Geometry check sheet. Reference: the model listing, model coordinates, mm. A direction names the side the tool comes from. Coordinates: 2 decimals unless noted, no trailing zeros. Write each loop counter-clockwise with the first axis right and the second up, starting at its lowest first coordinate (ties: lowest second). Pieces come first, ordered by that corner, then holes. Notation, with made-up numbers: M 85,60 L 142,60 A12 cw 142,66 Z; hole C 49,79.25 d8. An arc over 180 degrees is marked long. Put each result on its own line as item: value. Start each with the question number.
1) Set-up check for faces 1 (the flat face through (20, 3, 52)), 2 (the flat face through (2, 0, -45)), 3 (the cylindrical face through (22.11, 16.76, 45.33)): record each of +Z, -Z, +X, -X, +Y, -Y from which the full face is reachable in a straight line by a thin tool's end or side.
2) Cross-section at D-D on y = 17.5. Record the cut outline in (x, z).
3) Gauge pin test, flat ends, axial feed: pin 1 (6 mm diameter, centred on x = 22.5, z = 44.5, fed in from -Y); pin 2 (4 mm diameter, centred on x = 29.5, z = -41.5, fed in from +Y); pin 3 (3 mm diameter, centred on x = 4, y = 0, fed in from -Z); pin 4 (7.5 mm diameter, centred on x = 16, y = 0, fed in from -Z). Record the tip position at first contact, or that the pin passes through.
4) Mould release check, pull along X, two halves, no side actions. Record for faces 4 (the flat face through (16, 14, -40)), 5 (the flat face through (0, 0, -37)), 6 (the flat face through (32, 0, -18)): released by +X, released by -X, zero draft, split by the parting line, or undercut.
5) Cross-section at A-A on x = 4. Record the cut outline in (y, z).
6) Cross-section at B-B on z = -14. Record the cut outline in (x, y), plus the area to 3 significant figures.
7) Scan lines: line 1 along X through (y, z) = (0, -31); line 2 along Y through (x, z) = (16, -50); line 3 along Y through (x, z) = (4, -31.25). Record each from-to range of solid material in increasing order.
8) Cross-section at C-C on y = -25. Record the cut outline in (x, z).
from build123d import *

# Parameters (mm, degrees)
BOSS_EXTRUDE1_DEPTH       = 32
SKETCH4_R                 = 16
CUT_EXTRUDE3_DEPTH        = 15
SKETCH5_R                 = 7
SKETCH5_R_2               = 4
BOSS_EXTRUDE2_DEPTH       = 17
SKETCH15_W                = 16
SKETCH15_H                = 32
CUT_EXTRUDE6_DEPTH        = 15
SKETCH16_W                = 32
SKETCH16_H                = 32
BOSS_EXTRUDE6_DEPTH       = 30
SKETCH17_R                = 1.75
CUT_EXTRUDE8_DEPTH        = 53.92447449
CUT_EXTRUDE10_START       = -10
CUT_EXTRUDE10_DEPTH       = 5
SKETCH20_R                = 4.25
CUT_EXTRUDE11_DEPTH       = 39
CUT_EXTRUDE12_DEPTH       = 10
SKETCH22_R                = 6.5
CUT_EXTRUDE13_DEPTH       = 10
SKETCH23_R                = 1.75
CUT_EXTRUDE14_DEPTH       = 10
CUT_EXTRUDE16_REACH       = 64.498
SKETCH24_R                = 22.5
BOSS_EXTRUDE7_START       = 11.749999897
BOSS_EXTRUDE7_DEPTH       = 8.500000103
SKETCH26_R                = 8.5
CUT_EXTRUDE17_DEPTH       = 10
SKETCH27_R                = 16
BOSS_EXTRUDE8_DEPTH       = 7
SKETCH28_R                = 35
CUT_EXTRUDE18_DEPTH       = 63.498000008
BOSS_EXTRUDE9_START       = -7
SKETCH29_R                = 35
BOSS_EXTRUDE9_DEPTH       = 7
BOSS_EXTRUDE10_DEPTH      = 3
SKETCH31_R                = 15
CUT_EXTRUDE19_DEPTH       = 69.804069679
SKETCH32_R                = 2.2
CUT_EXTRUDE20_DEPTH       = 69.804069679
BOSS_EXTRUDE11_DEPTH      = 10
BOSS_EXTRUDE11_DEPTH_BACK = 10
SKETCH33_R                = 40
SKETCH33_R_2              = 29.5
CUT_EXTRUDE21_START       = -10
SKETCH34_R                = 29.5
CUT_EXTRUDE21_DEPTH       = 10
SKETCH35_W                = 26.144944591
SKETCH35_H                = 6
CUT_EXTRUDE22_DEPTH       = 71.887234394
SKETCH36_W                = 13.986084995
SKETCH36_H                = 10
BOSS_EXTRUDE12_DEPTH      = 20
CUT_EXTRUDE23_DEPTH       = 88.893005187
CUT_EXTRUDE23_DEPTH_BACK  = 88.893005187
SKETCH37_R                = 2.25
SKETCH38_R                = 5
CUT_EXTRUDE24_DEPTH       = 88.893005284
CUT_EXTRUDE25_DEPTH       = 88.893005284


# Read off the part's stored shape, not the designer's step: Boss-Extrude7
with BuildPart() as part:
    # Sketch1 → Boss-Extrude1 (new body)
    with BuildSketch(Plane(origin=(0, 0, 0), x_dir=(0, -1, 0), z_dir=(1, 0, 0))):
        with BuildLine():
            ThreePointArc((-16, 0), (0, 16), (16, 0))
            Line((16, 0), (16, 25))
            Line((16, 25), (-16, 25))
            Line((-16, 25), (-16, 0))
        make_face()
        with BuildLine():
            ThreePointArc((-4.5, 0), (0, 4.5), (4.5, 0))
            Line((4.5, 0), (16, 0))
            ThreePointArc((16, 0), (0, 16), (-16, 0))
            Line((-16, 0), (-4.5, 0))
        make_face()
        with BuildLine():
            Line((16, 0), (4.5, 0))
            ThreePointArc((4.5, 0), (0, -4.5), (-4.5, 0))
            Line((-4.5, 0), (-16, 0))
            ThreePointArc((-16, 0), (0, -16), (16, 0))
        make_face()
        with BuildLine():
            ThreePointArc((-4.5, 0), (0, 4.5), (4.5, 0))
            Line((4.5, 0), (16, 0))
            ThreePointArc((16, 0), (0, 16), (-16, 0))
            Line((-16, 0), (-4.5, 0))
        make_face()
        with BuildLine():
            Line((16, 0), (4.5, 0))
            ThreePointArc((4.5, 0), (0, -4.5), (-4.5, 0))
            Line((-4.5, 0), (-16, 0))
            ThreePointArc((-16, 0), (0, -16), (16, 0))
        make_face()
    extrude(amount=BOSS_EXTRUDE1_DEPTH)

    # Sketch4 → Cut-Extrude3 (cut)
    with BuildSketch(Plane.ZY):
        Circle(SKETCH4_R)
    extrude(amount=-CUT_EXTRUDE3_DEPTH, mode=Mode.SUBTRACT)

    # Sketch5 → Boss-Extrude2 (add)
    with BuildSketch(Plane.ZY.offset(-15)):
        Circle(SKETCH5_R)
        Circle(SKETCH5_R_2, mode=Mode.SUBTRACT)
    extrude(amount=-BOSS_EXTRUDE2_DEPTH)

    # Sketch15 → Cut-Extrude6 (cut)
    with BuildSketch(Plane.ZY):
        with Locations((-8, 0)):
            Rectangle(SKETCH15_W, SKETCH15_H)
    extrude(amount=-CUT_EXTRUDE6_DEPTH, mode=Mode.SUBTRACT)

    # Sketch16 → Boss-Extrude6 (add)
    with BuildSketch(Plane(origin=(0, 0, -25), x_dir=(-1, 0, 0), z_dir=(0, 0, -1))):
        with Locations((-16, 0)):
            Rectangle(SKETCH16_W, SKETCH16_H)
    extrude(amount=BOSS_EXTRUDE6_DEPTH)

    # Sketch17 → Cut-Extrude8 (cut, through all)
    with BuildSketch(Plane.XY.offset(-16)):
        with Locations((4, 0)):
            Circle(SKETCH17_R)
        with Locations((16, 12)):
            Circle(SKETCH17_R)
        with Locations((28, 0)):
            Circle(SKETCH17_R)
        with Locations((16, -12)):
            Circle(SKETCH17_R)
    extrude(amount=-CUT_EXTRUDE8_DEPTH, mode=Mode.SUBTRACT)

    # Sketch19 → Cut-Extrude10 (cut)
    with BuildSketch(Plane(origin=(0, 0, -55), x_dir=(-1, 0, 0), z_dir=(0, 0, -1)).offset(CUT_EXTRUDE10_START)):
        Polygon((0, 3), (-5.732050808, 3), (-7.464101615, 0), (-5.732050808, -3), (0, -3), align=None)
        Polygon((-16, -8.535898385), (-19, -10.267949192), (-19, -16), (-13, -16), (-13, -10.267949192), align=None)
        Polygon((-24.535898385, 0), (-26.267949192, 3), (-32, 3), (-32, -3), (-26.267949192, -3), align=None)
        Polygon((-16, 8.535898385), (-13, 10.267949192), (-13, 16), (-19, 16), (-19, 10.267949192), align=None)
    extrude(amount=-CUT_EXTRUDE10_DEPTH, mode=Mode.SUBTRACT)

    # Sketch20 → Cut-Extrude11 (cut)
    with BuildSketch(Plane(origin=(0, 0, -55), x_dir=(-1, 0, 0), z_dir=(0, 0, -1))):
        with Locations((-16, 0)):
            Circle(SKETCH20_R)
    extrude(amount=-CUT_EXTRUDE11_DEPTH, mode=Mode.SUBTRACT)

    # Sketch21 → Cut-Extrude12 (cut)
    with BuildSketch(Plane.ZY.offset(-15)):
        with BuildLine():
            Line((0, 16), (-16, 16))
            Line((-16, 16), (-16, 13.436140662))
            Line((-16, 13.436140662), (-16, 10.563859338))
            Line((-16, 10.563859338), (-16, 4.13067791))
            Line((-16, 4.13067791), (-16, -4.13067791))
            Line((-16, -4.13067791), (-16, -10.563859338))
            Line((-16, -10.563859338), (-16, -13.436140662))
            Line((-16, -13.436140662), (-16, -16))
            Line((-16, -16), (0, -16))
            ThreePointArc((0, -16), (16, 0), (0, 16))
        make_face()
    extrude(amount=-CUT_EXTRUDE12_DEPTH, mode=Mode.SUBTRACT)

    # Sketch22 → Cut-Extrude13 (cut)
    with BuildSketch(Plane.ZY.offset(-25)):
        Circle(SKETCH22_R)
    extrude(amount=-CUT_EXTRUDE13_DEPTH, mode=Mode.SUBTRACT)

    # Sketch23 → Cut-Extrude14 (cut)
    with BuildSketch(Plane.ZY.offset(-25)):
        with Locations((0, 12.5)):
            Circle(SKETCH23_R)
        with Locations((0, -12.5)):
            Circle(SKETCH23_R)
    extrude(amount=-CUT_EXTRUDE14_DEPTH, mode=Mode.SUBTRACT)

    # Cut-Extrude16: up to this face of the body (flat: up to its plane)
    cut_extrude16_end = Plane(part.part.faces().sort_by_distance((0, 0, -35.327586207))[0])
    # Sketch24 → Cut-Extrude16 (cut, up to the picked face)
    with BuildSketch(Plane.ZY.offset(-25), mode=Mode.PRIVATE) as cut_extrude16_sk1:
        Circle(SKETCH24_R)
    cut_extrude16_tool1 = split(extrude(cut_extrude16_sk1.sketch, amount=CUT_EXTRUDE16_REACH, mode=Mode.PRIVATE), bisect_by=cut_extrude16_end, keep=Keep.BOTH, mode=Mode.PRIVATE)
    add(cut_extrude16_tool1.solids().sort_by(Axis((25, 0, 0), (-1, 0, 0)))[0], mode=Mode.SUBTRACT)

    # Boss-Extrude7 outline → Boss-Extrude7 (add)
    with BuildSketch(Plane.YZ.offset(BOSS_EXTRUDE7_START)):
        with BuildLine():
            ThreePointArc((6, -21.685248442), (0, -22.5), (-6, -21.685248442))
            Line((-6, -21.685248442), (-6, -30))
            Line((-6, -30), (6, -30))
            Line((6, -30), (6, -21.685248442))
        make_face()
    extrude(amount=BOSS_EXTRUDE7_DEPTH)

    # Sketch26 → Cut-Extrude17 (cut)
    with BuildSketch(Plane.ZY.offset(-25)):
        Circle(SKETCH26_R)
    extrude(amount=-CUT_EXTRUDE17_DEPTH, mode=Mode.SUBTRACT)

    # Sketch27 → Boss-Extrude8 (add)
    with BuildSketch(Plane.ZY.offset(-25)):
        Circle(SKETCH27_R)
    extrude(amount=-BOSS_EXTRUDE8_DEPTH)

    # Sketch28 → Cut-Extrude18 (cut, through all)
    with BuildSketch(Plane.ZY.offset(-25)):
        with Locations((12.5, 0)):
            Circle(SKETCH28_R)
    extrude(amount=CUT_EXTRUDE18_DEPTH, mode=Mode.SUBTRACT)

    # Sketch29 → Boss-Extrude9 (add)
    with BuildSketch(Plane.ZY.offset(-25).offset(BOSS_EXTRUDE9_START)):
        with Locations((12.5, 0)):
            Circle(SKETCH29_R)
    extrude(amount=BOSS_EXTRUDE9_DEPTH)

    # Sketch30 → Boss-Extrude10 (add)
    with BuildSketch(Plane.ZY.offset(-25)):
        with BuildLine():
            ThreePointArc((-18.628764833, -16), (47.5, 0), (-18.628764833, 16))
            ThreePointArc((-18.628764833, 16), (-22.5, 0), (-18.628764833, -16))
        make_face()
    extrude(amount=BOSS_EXTRUDE10_DEPTH)

    # Sketch31 → Cut-Extrude19 (cut, through all)
    with BuildSketch(Plane.ZY.offset(-22)):
        with Locations((12.5, 0)):
            Circle(SKETCH31_R)
    extrude(amount=-CUT_EXTRUDE19_DEPTH, mode=Mode.SUBTRACT)

    # Sketch32 → Cut-Extrude20 (cut, through all)
    with BuildSketch(Plane.ZY.offset(-22)):
        with Locations((12.52327174, 25.399989339)):
            Circle(SKETCH32_R)
        with Locations((-5.444049099, 17.976960309)):
            Circle(SKETCH32_R)
        with Locations((-12.899989339, 0.02327174)):
            Circle(SKETCH32_R)
        with Locations((-5.476960309, -17.944049099)):
            Circle(SKETCH32_R)
        with Locations((12.47672826, -25.399989339)):
            Circle(SKETCH32_R)
        with Locations((30.444049099, -17.976960309)):
            Circle(SKETCH32_R)
        with Locations((30.476960309, 17.944049099)):
            Circle(SKETCH32_R)
    extrude(amount=-CUT_EXTRUDE20_DEPTH, mode=Mode.SUBTRACT)

    # Sketch33 → Boss-Extrude11 (add, two sides: drawn at the far end of the back side and taken through both)
    with BuildSketch(Plane.ZY.offset(-22).offset(-BOSS_EXTRUDE11_DEPTH_BACK)):
        with Locations((12.5, 0)):
            Circle(SKETCH33_R)
        with Locations((12.5, 0)):
            Circle(SKETCH33_R_2, mode=Mode.SUBTRACT)
    extrude(amount=BOSS_EXTRUDE11_DEPTH + BOSS_EXTRUDE11_DEPTH_BACK)

    # Sketch34 → Cut-Extrude21 (cut)
    with BuildSketch(Plane.ZY.offset(-22).offset(CUT_EXTRUDE21_START)):
        with Locations((12.5, 0)):
            Circle(SKETCH34_R)
    extrude(amount=CUT_EXTRUDE21_DEPTH, mode=Mode.SUBTRACT)

    # Sketch35 → Cut-Extrude22 (cut, through all)
    with BuildSketch(Plane.ZY.offset(-12)):
        with Locations((47.365138907, 0)):
            Rectangle(SKETCH35_W, SKETCH35_H)
    extrude(amount=-CUT_EXTRUDE22_DEPTH, mode=Mode.SUBTRACT)

    # Sketch36 → Boss-Extrude12 (add)
    with BuildSketch(Plane.ZY.offset(-12)):
        with Locations((55.394298853, 8)):
            Rectangle(SKETCH36_W, SKETCH36_H)
        with Locations((55.394298853, -8)):
            Rectangle(SKETCH36_W, SKETCH36_H)
    extrude(amount=-BOSS_EXTRUDE12_DEPTH)

    # Sketch37 → Cut-Extrude23 (cut, two sides: drawn at the far end of the back side and taken through both)
    with BuildSketch(Plane(origin=(0, 13, 0), x_dir=(1, 0, 0), z_dir=(0, 1, 0)).offset(-CUT_EXTRUDE23_DEPTH_BACK)):
        with Locations((22, -50.328560639)):
            Circle(SKETCH37_R)
    extrude(amount=CUT_EXTRUDE23_DEPTH + CUT_EXTRUDE23_DEPTH_BACK, mode=Mode.SUBTRACT)

    # Sketch38 → Cut-Extrude24 (cut, through all)
    with BuildSketch(Plane(origin=(0, 13, 0), x_dir=(1, 0, 0), z_dir=(0, 1, 0))):
        with Locations((22, -50.328560639)):
            Circle(SKETCH38_R)
    extrude(amount=CUT_EXTRUDE24_DEPTH, mode=Mode.SUBTRACT)

    # Sketch39 → Cut-Extrude25 (cut, through all)
    with BuildSketch(Plane.XZ.offset(13)):
        Polygon((25.75, 52.493624148), (22, 54.658687658), (18.25, 52.493624148), (18.25, 48.163497129), (22, 45.99843362), (25.75, 48.163497129), align=None)
    extrude(amount=CUT_EXTRUDE25_DEPTH, mode=Mode.SUBTRACT)


solid = part.part
Answer key:
1. face 1: +Z, +X, -X
1. face 2: -X
1. face 3: +Z, +Y
2. outline: M 12,-23.47 L 32,-23.47 L 32,-11.25 L 12,-11.25 Z; M 12,36.25 L 32,36.25 L 32,48.47 L 26.64,48.47 A5 cw 17.36,48.47 L 12,48.47 Z
3. pin 1: stops at y = -27.55
3. pin 2: stops at y = 16
3. pin 3: passes through
3. pin 4: stops at z = -30
4. face 4: undercut
4. face 5: released by -X
4. face 6: released by +X
5. outline: M -16,-55 L -1.75,-55 L -1.75,-45 L -3,-45 L -3,-40 L -1.75,-40 L -1.75,-22.46 A35 cw -16,-18.63 Z; M 1.75,-55 L 16,-55 L 16,-18.63 A35 cw 1.75,-22.46 L 1.75,-40 L 3,-40 L 3,-45 L 1.75,-45 Z
6. outline: M 12,-29.96 L 32,-29.96 L 32,-12.96 L 12,-12.96 Z; M 12,12.96 L 32,12.96 L 32,29.96 L 12,29.96 Z
6. area: 680 mm²
7. line 1: x = 0 to 2.25, 5.75 to 11.75, 20.25 to 26.25, 29.75 to 32
7. line 2: y = -16 to -13.75, -10.25 to -4.25, 4.25 to 10.25, 13.75 to 16
7. line 3: y = -16 to -1.75, 1.75 to 16
8. outline: M 12,-18.72 L 32,-18.72 L 32,-3.16 L 12,-3.16 Z; M 12,28.16 L 32,28.16 L 32,43.72 L 12,43.72 Z
